Geometry: see drawing. Coordinates: mm, zero at the bounding-box minimum. A direction names the side the tool comes from. Give positions to 0.01 mm unless a question says otherwise; leave off trailing zeros. Loops run counter-clockwise (first coordinate to the right, second up) from the corner with the lowest first, then second, coordinate; pieces in that order, holes last. Notation, with made-up numbers: M 25.25,57.5 L 29.25,57.5 A35 ccw 29.25,89.5 Z; hole C 14.5,44 d2. An arc over 180 degrees is marked long. Return JSON: item names as keys, results as strings. Group by question number.
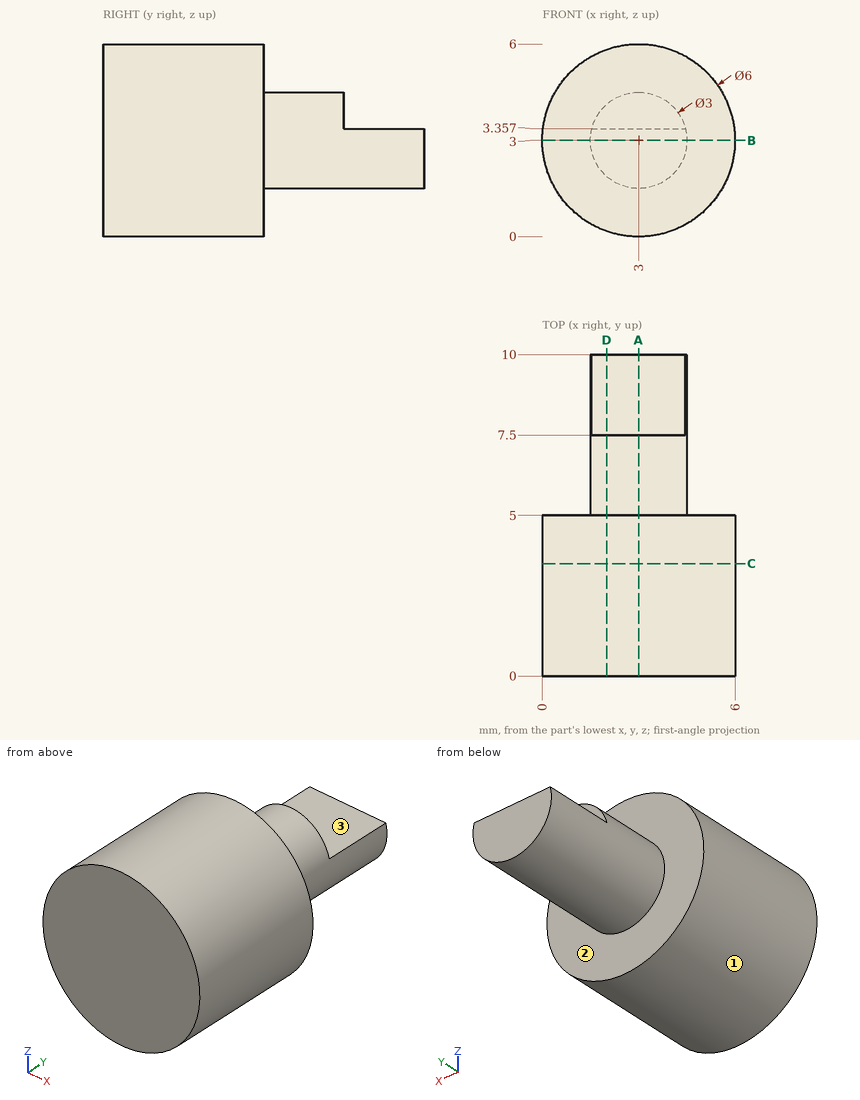
Item 1: Material intervals for line 1 (Y direction, x = 4, z = 3.7); line 2 (Z direction, x = 3.1, y = 3.5); line 3 (Z direction, x = 2.65, y = 6.75), sorted ascending. Write a range as from..to.
Item 2: Reachability of the marked faces 1, 2 and 3 from +Z, -Z, +X, -X, +Y, -Y: full face, straight path, thin tool, end or side. Return the list, or none.
Item 3: Section C-C, the plane y = 3.5. Return loops of the section in (x, z), then the cut area to 3 significant figures.
Item 4: First-contact query: pin 1 Ø3 at (y, z) = (7.5, 1.5) entering from +X. Flat tip, straight axial feed; report the tip coordinate or a pass-through.
Item 5: Section A-A, the plane x = 3. Return loops of the section in (y, z).
Item 6: Section D-D, the plane x = 2. Return loops of the section in (y, z).
Item 7: Section B-B, the plane z = 3. Return loops of the section in (x, y), then the cut area to 3 significant figures.
Answer below:
{
 "1": {"line 1": "0..7.5", "line 2": "0..6", "line 3": "1.54..4.46"},
 "2": {"face 1": "+Y, -Y", "face 2": "+Y", "face 3": "+Z, +X, -X, +Y"},
 "3": {"outline": "C 3,3 d6", "area": "28.3 mm^2"},
 "4": {"pin 1": "x = 4.5"},
 "5": {"outline": "M 0,0 L 5,0 L 5,1.5 L 10,1.5 L 10,3.36 L 7.5,3.36 L 7.5,4.5 L 5,4.5 L 5,6 L 0,6 Z"},
 "6": {"outline": "M 0,0.17 L 5,0.17 L 5,1.88 L 10,1.88 L 10,3.36 L 7.5,3.36 L 7.5,4.12 L 5,4.12 L 5,5.83 L 0,5.83 Z"},
 "7": {"outline": "M 0,0 L 6,0 L 6,5 L 4.5,5 L 4.5,10 L 1.5,10 L 1.5,5 L 0,5 Z", "area": "45.0 mm^2"}
}
